Can you work these out from the model? Positions are in its coordinate system, mm. A direction names the side the tool comes from. Round coordinates to 2 decimals unless told otherwise and drop trailing zeros. Order: outer loops, then holes, each group sorted by start corner. A loop starts at its lowest first (then second) coordinate and runs counter-clockwise, first axis right, second up. Notation, with made-up numbers: (40.5, 74.25) -> (95.5, 74.25) arc R17 ccw to (95.5, 80.25) -> close; hole circle Ø10 at (60, 50.5). An arc over 180 degrees is marked (long way). Use a Markdown table: item, result. Add a question column.
Q1. I'm going to push flat-ended pins straight in: pin 1 Ø2 at (y, z) = (2, -4) entering from +X; pin 2 Ø6.5 at (x, z) = (0.5, -2) entering from -Y; pin 3 Ø5.5 at (x, z) = (0, 0) entering from +Y. Where does each tip first touch, or does it pass through?
Q2. We'd pull the mould along Z, two halves only. Please class faces 4 (the face through (3, 6.061, 4)), 5 (the face through (6.694, 5.407, -0.295)), 6 (the face through (0.45, 2.66, -3.42)): +Z half, -Z half, draft (parallel to the pull), parting line (faces both ways), or undercut.
Q3. For faces 1 (the face through (-1, 0, 4)), 2 (the face through (0, 5.061, 6)), 3 (the face through (-5.256, 4.183, -1.655)), which set-ups out of +Z, -Z, +X, -X, +Y, -Y let a thin tool reach every point of the face, with its end or its side?
Q4. I need wall thicknesses on line 1 along X through (y, z) = (2.1, 0); line 2 along Z through (x, y) = (0, 4). Which ranges of each line are inside material? Lowest first, please. Write a range as [from, to].
Q5. If we section it at B-B on y = 2.5: List the corners of the cut face in (x, z) for me, plus the area to 3 significant figures.
Q6. If we section it at A-A on y = 4: List the corners of the cut face in (x, z) for me, plus the area to 3 significant figures.
```python
from build123d import *


with BuildPart() as part:
    # Sketch1 → Main Revolve (revolve)
    with BuildSketch(Plane.XY):
        with BuildLine():
            ThreePointArc((-3.65, 0), (-3.508578644, 0.058578644), (-3.45, 0.2))
            Line((-3.45, 0.2), (-3.45, 5.060607))
            ThreePointArc((-3.45, 5.060607), (-3.742893219, 5.767713781), (-4.45, 6.060607))
            Line((-4.45, 6.060607), (-6.3, 6.060607))
            Line((-6.3, 6.060607), (-6.7, 5.660607))
            Line((-6.7, 5.660607), (-6.7, 5.160607))
            Line((-6.7, 5.160607), (-6.6, 5.060607))
            Line((-6.6, 5.060607), (-5.81, 5.060607))
            ThreePointArc((-5.81, 5.060607), (-5.597867966, 4.972739034), (-5.51, 4.760607))
            Line((-5.51, 4.760607), (-5.51, 3.6214998))
            ThreePointArc((-5.51, 3.6214998), (-5.522579117, 3.463385917), (-5.56, 3.3092499))
            ThreePointArc((-5.56, 3.3092499), (-5.597420883, 3.155113883), (-5.61, 2.997))
            Line((-5.61, 2.997), (-5.61, 0.2))
            ThreePointArc((-5.61, 0.2), (-5.551421356, 0.058578644), (-5.41, 0))
            Line((-5.41, 0), (-3.65, 0))
        make_face()
    revolve(axis=Axis((0, 11.984375, 0), (0, -1, 0)))


solid = part.part
```
Answer below:
| question | item | result |
|---|---|---|
| 1 | pin 1 | x = 4.74 |
| 1 | pin 2 | y = 0 |
| 1 | pin 3 | through |
| 2 | face 4 | draft |
| 2 | face 5 | parting line |
| 2 | face 6 | undercut |
| 3 | face 1 | +Z, -Z, +X, -X, -Y |
| 3 | face 2 | -Y |
| 3 | face 3 | none |
| 4 | line 1 | [-5.61, -3.45], [3.45, 5.61] |
| 4 | line 2 | [-5.51, -3.45], [3.45, 5.51] |
| 5 | outline | circle Ø11.22 at (0, 0); hole circle Ø6.9 at (0, 0) |
| 5 | area | 61.5 mm² |
| 6 | outline | circle Ø11.02 at (0, 0); hole circle Ø6.9 at (0, 0) |
| 6 | area | 58.0 mm² |
